Geometry: see drawing. Coordinates: mm, zero at the bounding-box minimum. A direction names the side the tool comes from. Give positions to 0.01 mm unless a question says otherwise; leave off trailing zeros. Loops run counter-clockwise (first coordinate to the right, second up) from the corner with the lowest first, then second, coordinate; pieces in that order, holes last. Notation, with made-up numbers: (-34, 39) -> (19, 39) arc R18 ccw to (19, 63) -> close; hole circle Ø9 at (0.5, -38.75). An arc over 180 degrees is marked (long way). One line per question, with ' | ' between items.
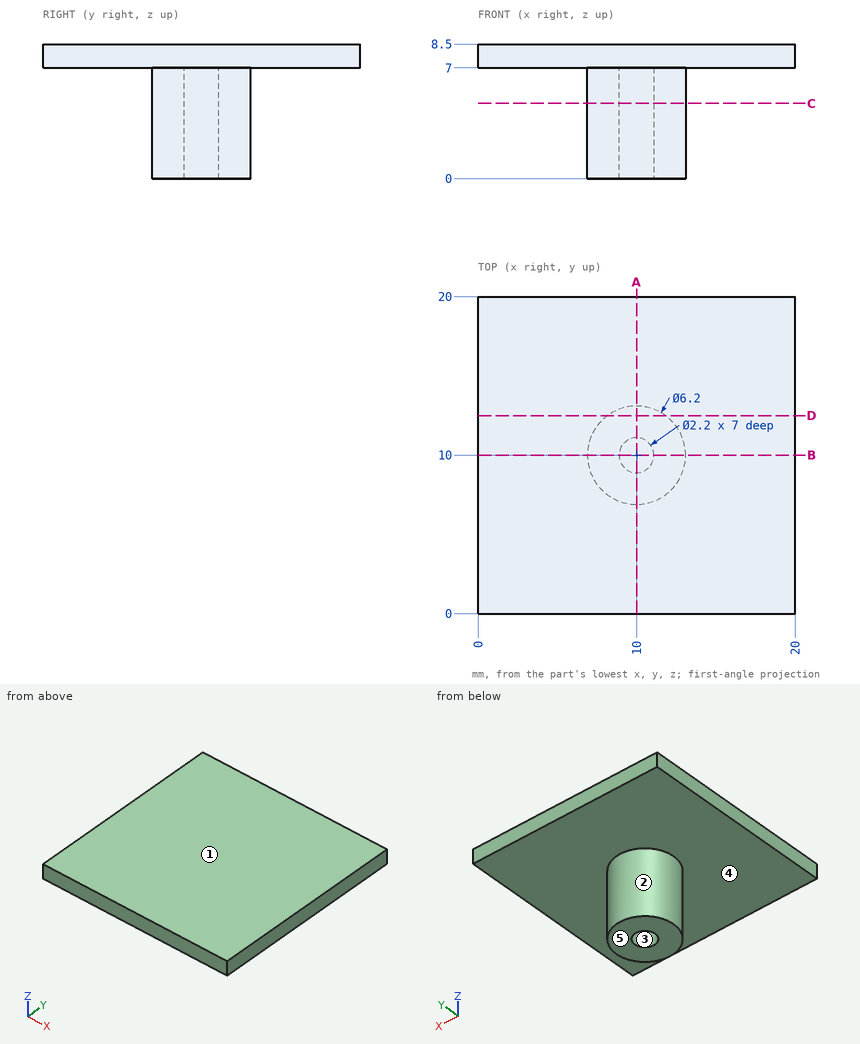
1. Reachability of the marked faces 4 and 5 from +Z, -Z, +X, -X, +Y, -Y: full face, straight path, thin tool, end or side. Return the list, or none.
Determined:
face 4: -Z | face 5: -Z, +X, -X, +Y, -Y
2. Section query C-C (z = 4.75). Output: boundary loops of the cut face in (x, y), then the cut area to 3 significant figures.
Determined:
outline: circle Ø6.2 at (10, 10); hole circle Ø2.2 at (10, 10) | area: 26.4 mm2
3. Ray query, line 1 along Y through (x, z) = (10, 4.75); line 2 along Z through (x, y) = (8.75, 17.5); line 3 along Y through (x, z) = (9.5, 4.75). Return the intervals inside material, ascending. Write a range as from..to.
Determined:
line 1: y = 6.9..8.9, 11.1..13.1 | line 2: z = 7..8.5 | line 3: y = 6.94..9.02, 10.98..13.06
4. Pull-direction query (Y, two-part tool) for the marked faces 1, 2 and 3; classes: pulls with the +Y half, pulls with the -Y half, needs draft (parallel to the pull), parting line crosses it, or undercut.
Determined:
face 1: needs draft | face 2: parting line crosses it | face 3: undercut
5. Section query A-A (x = 10). Output: boundary loops of the cut face in (y, z).
Determined:
outline: (0, 7) -> (6.9, 7) -> (6.9, 0) -> (8.9, 0) -> (8.9, 7) -> (11.1, 7) -> (11.1, 0) -> (13.1, 0) -> (13.1, 7) -> (20, 7) -> (20, 8.5) -> (0, 8.5) -> close
6. Section query D-D (y = 12.5). Output: boundary loops of the cut face in (x, z).
Determined:
outline: (0, 7) -> (8.17, 7) -> (8.17, 0) -> (11.83, 0) -> (11.83, 7) -> (20, 7) -> (20, 8.5) -> (0, 8.5) -> close
7. Pin query (flat end, axial travel): P1, Ø1, axis at y = 14.5, z = 3.5, coming from the -X side; P2, Ø0.7, axis at x = 10, y = 10.5, coming from the -Z side; P3, Ø1.5, axis at y = 13, z = 5.5, coming from the +X side. Return the tip coordinate at first contact, or that it passes through.
Determined:
P1: passes through | P2: stops at z = 7 | P3: stops at x = 12.13
